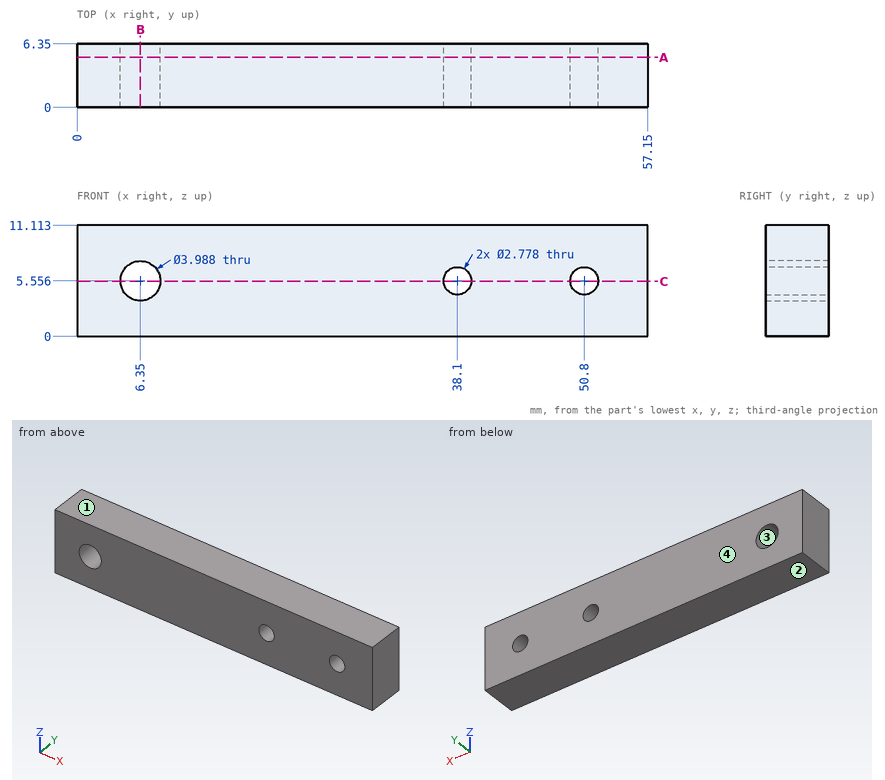
Here's the drawing with two shaded views (mm, measured from the low corner). I have some questions. Round coordinates to 2 decimals unless told otherwise and drop trailing zeros. Write each loop counter-clockwise with the first axis right and the second up, starting at its lowest first coordinate (ties: lowest second). Pieces come first, ordered by that corner, then holes. Notation, with made-up numbers: M 19.5,71 L 47.5,71 A10 ccw 47.5,87 Z; hole C 25,8.25 d9. An arc over 180 degrees is marked long. Use CSV: the item, a comma, the result in double quotes.
(1) I'm going to push a flat-ended pin straight in: pin 1 (3.5 mm diameter, centred on x = 6.35, z = 5.56, fed in from +Y). Where does the tip first touch, or does it pass through?
Check values:
pin 1,"through"
(2) Imagine slicing it at B-B (x = 6.35). Write out the boundary of the cut face in (y, z).
Check values:
outline,"M 0,0 L 6.35,0 L 6.35,3.56 L 0,3.56 Z; M 0,7.55 L 6.35,7.55 L 6.35,11.11 L 0,11.11 Z"
(3) We'd pull the mould along Z, two halves only. Please class the marked faces 1, 2, 3 and 4: +Z half, -Z half, draft (parallel to the pull), parting line (faces both ways), or undercut.
Check values:
face 1,"+Z half"
face 2,"-Z half"
face 3,"undercut"
face 4,"draft"
(4) Imagine slicing it at A-A (y = 5). Count the separate pieces of the cut face and the enclosed holes in it.
Check values:
separate pieces,"1"
enclosed holes,"3"
(5) Imagine slicing it at C-C (z = 5.5). Write out the boundary of the cut face in (x, y).
Check values:
outline,"M 0,0 L 4.36,0 L 4.36,6.35 L 0,6.35 Z; M 8.34,0 L 36.71,0 L 36.71,6.35 L 8.34,6.35 Z; M 39.49,0 L 49.41,0 L 49.41,6.35 L 39.49,6.35 Z; M 52.19,0 L 57.15,0 L 57.15,6.35 L 52.19,6.35 Z"
